Verification items for this drawing (mm, ordinates from the low corner). Coordinates: 2 decimals unless noted, no trailing zeros. Order: outer loops, then holes, each group sorted by start corner. A loop starts at its lowest first (then second) coordinate and runs counter-clockwise, first axis right, second up.
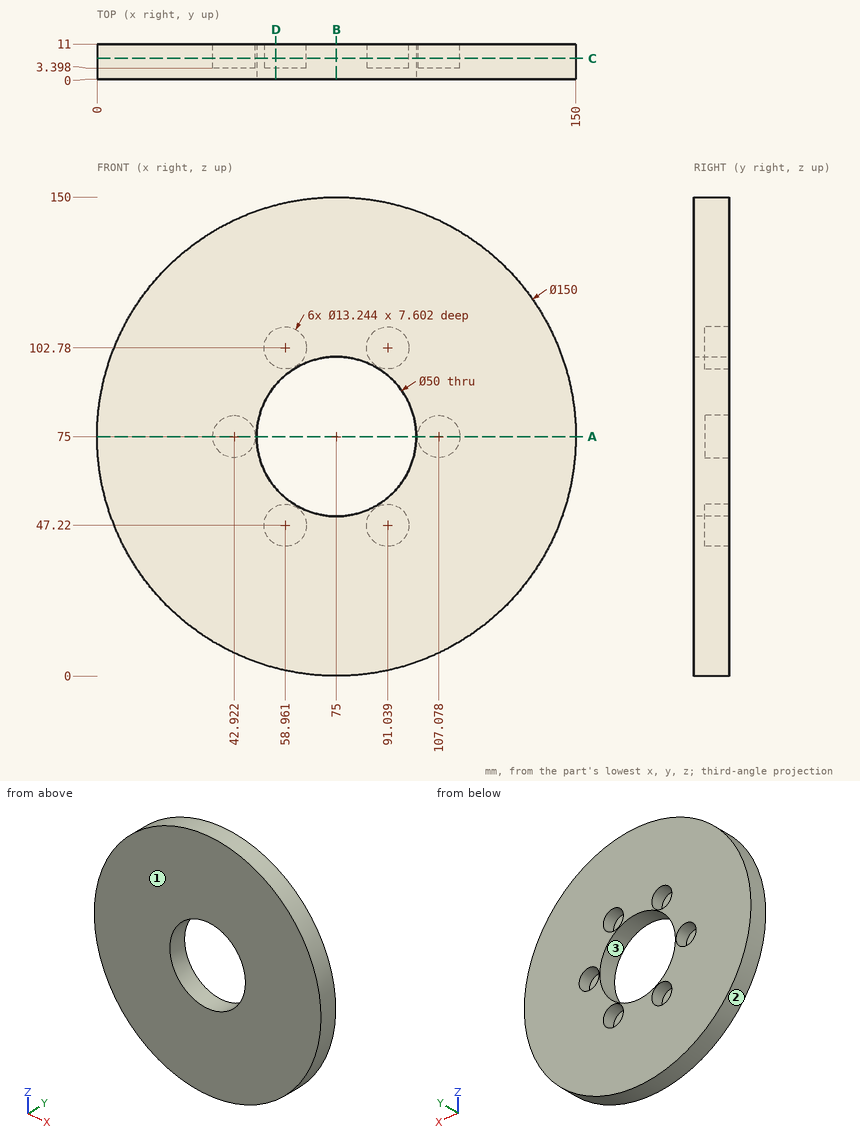
(1) Go/stop test with flat-tipped pins: P1, Ø10.5, axis at x = 90.5, z = 47, coming from the +Y side; P2, Ø1.5, axis at x = 108, y = 5.5, coming from the -Z side; P3, Ø1.5, axis at x = 90.5, y = 4.5, coming from the -Z side (1 decimal). Record where each tip stops, or that it passes through.
Filled in:
P1: stops at y = 3.4
P2: stops at z = 7.29
P3: stops at z = 1.5
(2) Release check for a two-part mould opening along X. For the marked faces 1, 2 and 3 record: +X half, -X half, draft (parallel to the pull), parting line (faces both ways), or undercut.
Filled in:
face 1: draft
face 2: parting line
face 3: undercut
(3) Cross-section at B-B (x = 75). Enter the section's corners in (y, z).
Filled in:
outline: (0, 0) - (11, 0) - (11, 50) - (0, 50) - close; (0, 100) - (11, 100) - (11, 150) - (0, 150) - close
(4) Thickness scan on probe 1 along X at (y, z) = (9, 75); probe 2 along Z at (x, y) = (97, 9.5) (1 decimal); probe 3 along Z at (x, y) = (91, 9.5) (1 decimal). Record the ranges inside material, lowest first.
Filled in:
probe 1: x = 0 to 36.3, 49.54 to 50, 100 to 100.46, 113.7 to 150
probe 2: z = 3.3 to 44.3, 50.1 to 63.1, 86.9 to 99.9, 105.7 to 146.7
probe 3: z = 1.7 to 40.6, 53.8 to 55.8, 94.2 to 96.2, 109.4 to 148.3
(5) Cross-section at D-D (x = 56). Enter the section's corners in (y, z).
Filled in:
outline: (0, 2.45) - (11, 2.45) - (11, 41.3) - (3.4, 41.3) - (3.4, 53.14) - (11, 53.14) - (11, 58.75) - (0, 58.75) - close; (0, 91.25) - (11, 91.25) - (11, 96.86) - (3.4, 96.86) - (3.4, 108.7) - (11, 108.7) - (11, 147.55) - (0, 147.55) - close
(6) Cross-section at A-A (z = 75). Enter the section's corners in (x, y).
Filled in:
outline: (0, 0) - (50, 0) - (50, 11) - (49.54, 11) - (49.54, 3.4) - (36.3, 3.4) - (36.3, 11) - (0, 11) - close; (100, 0) - (150, 0) - (150, 11) - (113.7, 11) - (113.7, 3.4) - (100.46, 3.4) - (100.46, 11) - (100, 11) - close
(7) Cross-section at C-C (y = 6.5). Enter the section's corners in (x, z).
Filled in:
outline: circle Ø150 at (75, 75); hole circle Ø13.24 at (42.92, 75); hole circle Ø50 at (75, 75); hole circle Ø13.24 at (58.96, 47.22); hole circle Ø13.24 at (58.96, 102.78); hole circle Ø13.24 at (91.04, 47.22); hole circle Ø13.24 at (91.04, 102.78); hole circle Ø13.24 at (107.08, 75)
